from build123d import *

# Parameters (mm, degrees)
SALIENTE_EXTRUIR1_DEPTH = 22
CROQUIS4_R              = 1.75
CORTAR_EXTRUIR1_DEPTH   = 56.172456897
CROQUIS5_R              = 1.75
CORTAR_EXTRUIR2_DEPTH   = 54.058929503
REDONDEO1_R             = 6
REDONDEO2_R             = 5
REDONDEO3_R             = 1.5
SALIENTE_EXTRUIR2_START = 3
CROQUIS6_R              = 3.5
CROQUIS6_R_2            = 1.75
SALIENTE_EXTRUIR2_DEPTH = 3


with BuildPart() as part:
    # Croquis3 → Saliente-Extruir1 (new, symmetric)
    with BuildSketch(Plane(origin=(0, 0, 0), x_dir=(0, 0, -1), z_dir=(1, 0, 0))):
        Polygon((-11.5, 0), (-11.5, 3), (-1.5, 3), (-1.5, 48), (1.5, 48), (1.5, 3), (17.5, 3), (17.5, 0), (0, 0), align=None)
    extrude(amount=SALIENTE_EXTRUIR1_DEPTH, both=True)

    # Croquis4 → Cortar-Extruir1 (cut, through all)
    with BuildSketch(Plane(origin=(0, 0, -1.5), x_dir=(-1, 0, 0), z_dir=(0, 0, -1))):
        with Locations(Location((15.5, 42.5, 0), (0, 0, 90))):
            Circle(CROQUIS4_R)
        with Locations(Location((-15.5, 11.5, 0), (0, 0, 90))):
            Circle(CROQUIS4_R)
    cortar_extruir1 = extrude(amount=-CORTAR_EXTRUIR1_DEPTH, mode=Mode.SUBTRACT)

    # Simetría1: Cortar-Extruir1 across plane
    add(cortar_extruir1.mirror(Plane(origin=(0, 0, 0), x_dir=(0, 0, 1), z_dir=(1, 0, 0))), mode=Mode.SUBTRACT)

    # Croquis5 → Cortar-Extruir2 (cut, through all)
    with BuildSketch(Plane(origin=(0, 3, 0), x_dir=(1, 0, 0), z_dir=(0, 1, 0))):
        with Locations(Location((-12, -6.5, 0), (0, 0, 270))):
            Circle(CROQUIS5_R)
        with Locations(Location((12, -6.5, 0), (0, 0, 270))):
            Circle(CROQUIS5_R)
    extrude(amount=-CORTAR_EXTRUIR2_DEPTH, mode=Mode.SUBTRACT)

    # Redondeo1
    redondeo1_edges = [part.edges().sort_by_distance(p)[0] for p in [
        (-22, 48, 0),
        (22, 48, 0),
    ]]
    fillet(redondeo1_edges, radius=REDONDEO1_R)

    # Redondeo2
    redondeo2_edges = [part.edges().sort_by_distance(p)[0] for p in [
        (-22, 1.5, 11.5),
        (-22, 1.5, -17.5),
        (22, 1.5, 11.5),
        (22, 1.5, -17.5),
    ]]
    fillet(redondeo2_edges, radius=REDONDEO2_R)

    # Redondeo3
    redondeo3_edges = [part.edges().sort_by_distance(p)[0] for p in [
        (0, 3, 1.5),
        (0, 3, -1.5),
    ]]
    fillet(redondeo3_edges, radius=REDONDEO3_R)

    # Croquis6 → Saliente-Extruir2 (add)
    # profile 1 of 2: a face of its own
    with BuildSketch(Plane(origin=(0, 0, -1.5), x_dir=(-1, 0, 0), z_dir=(0, 0, -1)).offset(SALIENTE_EXTRUIR2_START)):
        with Locations(Location((-15.5, 42.5, 0), (0, 0, 270))):
            Circle(CROQUIS6_R)
        with Locations(Location((-15.5, 42.5, 0), (0, 0, 90))):
            Circle(CROQUIS6_R_2, mode=Mode.SUBTRACT)
    # profile 2 of 2: a face of its own
    with BuildSketch(Plane(origin=(0, 0, -1.5), x_dir=(-1, 0, 0), z_dir=(0, 0, -1)).offset(SALIENTE_EXTRUIR2_START)):
        with Locations(Location((-15.5, 11.5, 0), (0, 0, 270))):
            Circle(CROQUIS6_R)
        with Locations(Location((-15.5, 11.5, 0), (0, 0, 90))):
            Circle(CROQUIS6_R_2, mode=Mode.SUBTRACT)
    saliente_extruir2 = extrude(amount=-SALIENTE_EXTRUIR2_DEPTH)

    # Simetría2: Saliente-Extruir2 across plane
    add(saliente_extruir2.mirror(Plane(origin=(0, 0, 0), x_dir=(0, 0, 1), z_dir=(1, 0, 0))))


solid = part.part
For this review, take the finished solid that the model builds, in its own axes (mm). A direction names the side the tool comes from. Give positions to 0.01 mm unless a question says otherwise; leave off trailing zeros. Write each loop counter-clockwise with the first axis right and the second up, starting at its lowest first coordinate (ties: lowest second). Pieces come first, ordered by that corner, then holes. Notation, with made-up numbers: (37, 79.5) -> (83, 79.5) arc R21 cw to (83, 97.5) -> close; hole circle Ø2 at (-15.75, -20). An arc over 180 degrees is marked (long way). Use CSV: the item, a comma, the result in double quotes.
Q1. Take a section at C-C, the plane z = -11. Write out the cut boundary in (x, y).
Conclusion:
outline,"(-22, 0) -> (22, 0) -> (22, 3) -> (-22, 3) -> close"
Q2. To check wall thickness, follow probe 1 along X at (y, z) = (11.5, -3); probe 2 along X at (y, z) = (11.5, -0.1); probe 3 along Y at (x, z) = (-17, -0.5). State the ranges of each line that lie inside material, in increasing order. Write a range as [from, to].
Conclusion:
probe 1,"[-19, -17.25], [-13.75, -12], [12, 13.75], [17.25, 19]"
probe 2,"[-22, -17.25], [-13.75, 13.75], [17.25, 22]"
probe 3,"[0, 10.6], [12.4, 41.6], [43.4, 47.92]"
Q3. Tool access review of faces 4 (the face through (-17, 10, -4.5)), 5 (the face through (-17.6, 14.3, -3)), 6 (the face through (-0.31, 3.43, 1.95)): name each direction out of +Z, -Z, +X, -X, +Y, -Y from which nothing blocks a thin tool from reaching the whole face with its end or side.
Conclusion:
face 4,"-Z, +X, -X, +Y"
face 5,"-Z"
face 6,"+Z, +X, -X, +Y"
Q4. For P1, Ø2, axis at x = -17, y = 13, coming from the -Z side; P2, Ø2, axis at x = -11.5, y = 13, coming from the +Z side; P3, Ø16, axis at x = -1.5, z = -11.5, coming from the +Y side; P4, Ø6, axis at x = -3, z = -7.5, coming from the -Y side, all flat-tipped, find the tip position at first contact; note any pin that passes through.
Conclusion:
P1,"z = -4.5"
P2,"z = 1.5"
P3,"y = 3"
P4,"y = 0"
Q5. Take a section at D-D, the plane y = 25. Write out the cut boundary in (x, z).
Conclusion:
outline,"(-22, -1.5) -> (22, -1.5) -> (22, 1.5) -> (-22, 1.5) -> close"
Q6. Mouldability with a two-part tool opening along Y and no side actions: class faces 1 (the face through (-17, 41, -4.5)), 2 (the face through (-0.31, 3.45, -1.93)), 3 (the face through (0, 0, -3)) as pulls with the +Y half, pulls with the -Y half, needs draft (parallel to the pull), parting line crosses it, or undercut.
Conclusion:
face 1,"needs draft"
face 2,"undercut"
face 3,"pulls with the -Y half"
Q7. Take a section at A-A, the plane y = 11.5. Write out the cut boundary in (x, z).
Conclusion:
outline,"(-22, -1.5) -> (-19, -1.5) -> (-19, -4.5) -> (-17.25, -4.5) -> (-17.25, 1.5) -> (-22, 1.5) -> close; (-13.75, -4.5) -> (-12, -4.5) -> (-12, -1.5) -> (12, -1.5) -> (12, -4.5) -> (13.75, -4.5) -> (13.75, 1.5) -> (-13.75, 1.5) -> close; (17.25, -4.5) -> (19, -4.5) -> (19, -1.5) -> (22, -1.5) -> (22, 1.5) -> (17.25, 1.5) -> close"
Q8. Take a section at B-B, the plane z = 7.25. Write out the cut boundary in (x, y).
Conclusion:
outline,"(-21.94, 0) -> (-13.58, 0) -> (-13.58, 3) -> (-21.94, 3) -> close; (-10.42, 0) -> (10.42, 0) -> (10.42, 3) -> (-10.42, 3) -> close; (13.58, 0) -> (21.94, 0) -> (21.94, 3) -> (13.58, 3) -> close"
